Source: CAD feature listing. Evaluate the final solid. Frame: model axes, mm. A direction names the side the tool comes from. Coordinates: 2 decimals unless noted, no trailing zeros. Write each loop counter-clockwise with the first axis right and the second up, starting at its lowest first coordinate (ties: lowest second). Pieces come first, ordered by that corner, then holes. Notation, with made-up numbers: (5.25, -2.5) - (47.25, -2.5) arc R14 cw to (47.25, 1.5) - close; hole circle Ø1 at (22, 66.5). An arc over 180 degrees is marked (long way). One line per question, with ' | ' between items. Start each with the question number.
Q1. Cut plane A-A, the plane y = 14.5. Return loops of the section in (x, z), plus the area to 3 significant figures.
Q2. Draft query along Z for faces 5 (the face through (-20, 51, 15)), 6 (the face through (15, 37, 20)), 7 (the face through (0, 50, 0)), 8 (the face through (12.5, 25, 16)). Return one class per face: +Z half, -Z half, draft (parallel to the pull), parting line (faces both ways), or undercut.
Q3. Access query for faces 1 (the face through (10, 63, -5)), 2 (the face through (-20.5, 25, 0)), 3 (the face through (10.2, 60.5, -7.5)), 4 (the face through (15, 37, -20)). Directions: +Z, -Z, +X, -X, +Y, -Y. A direction counts if a zero-diameter tool reaches every point of the face in a straight line with its end or side. Return the directions, or none.
Q4. Line query: line 1 (X direction, y = 3.5, z = 20); line 2 (X direction, y = 19, z = 0). Output: solid intervals per line, ascending.
Q5. Cut plane C-C, the plane x = -0.5. Return loops of the section in (y, z).
Q6. Contact query for flat-ended pins moving along their axis: P1, Ø5, axis at y = 23.5, z = -18, coming from the +X side; P2, Ø8, axis at x = 21, y = 37.5, coming from the -Z side; P3, Ø2, axis at x = -17.5, z = 4.5, coming from the -Y side; P4, Ø3, axis at y = 20.5, z = 16, coming from the -X side. Output: stop coordinate, or through.
Q7. Cut plane B-B, the plane z = 14. Return loops of the section in (x, y), plus the area to 3 significant figures.
Q8. Cut plane D-D, the plane y = 61. Return loops of the section in (x, z), plus the area to 3 significant figures.
```python
from build123d import *

# Parameters (mm, degrees)
SKETCH1_W           = 50
SKETCH1_H           = 50
BOSS_EXTRUDE1_DEPTH = 64
SKETCH2_W           = 10
SKETCH2_H           = 10
CUT_EXTRUDE1_DEPTH  = 55
CUT_EXTRUDE2_DEPTH  = 30
SKETCH4_W           = 10
SKETCH4_H           = 30
BOSS_EXTRUDE2_DEPTH = 30
SKETCH6_W           = 8
SKETCH6_H           = 25
SKETCH6_W_2         = 25
SKETCH6_H_2         = 8
CUT_EXTRUDE4_DEPTH  = 50
SKETCH7_R           = 3.6
CUT_EXTRUDE5_DEPTH  = 50
SKETCH8_R           = 2.65
CUT_EXTRUDE6_DEPTH  = 50


with BuildPart() as part:
    # Sketch1 → Boss-Extrude1 (new body)
    with BuildSketch(Plane(origin=(0, 0, 0), x_dir=(1, 0, 0), z_dir=(0, 1, 0))):
        Rectangle(SKETCH1_W, SKETCH1_H)
    extrude(amount=BOSS_EXTRUDE1_DEPTH)

    # Sketch2 → Cut-Extrude1 (cut)
    with BuildSketch(Plane(origin=(0, 64, 0), x_dir=(1, 0, 0), z_dir=(0, 1, 0))):
        with Locations((20, 20)):
            Rectangle(SKETCH2_W, SKETCH2_H)
        with Locations((-20, 20)):
            Rectangle(SKETCH2_W, SKETCH2_H)
        with Locations((20, -20)):
            Rectangle(SKETCH2_W, SKETCH2_H)
        with Locations((-20, -20)):
            Rectangle(SKETCH2_W, SKETCH2_H)
    extrude(amount=-CUT_EXTRUDE1_DEPTH, mode=Mode.SUBTRACT)

    # Sketch3 → Cut-Extrude2 (cut)
    with BuildSketch(Plane(origin=(25, 0, 0), x_dir=(0, 0, -1), z_dir=(1, 0, 0))):
        Polygon((-5, 64), (5, 64), (5, 62), (10, 59), (10, 57), (-10, 57), (-10, 59), (-5, 62), align=None)
    extrude(amount=-CUT_EXTRUDE2_DEPTH, mode=Mode.SUBTRACT)

    # Sketch4 → Boss-Extrude2 (add)
    with BuildSketch(Plane(origin=(0, 64, 0), x_dir=(1, 0, 0), z_dir=(0, 1, 0))):
        with Locations((-20, 0)):
            Rectangle(SKETCH4_W, SKETCH4_H)
    extrude(amount=BOSS_EXTRUDE2_DEPTH)

    # Sketch6 → Cut-Extrude4 (cut)
    with BuildSketch(Plane.XZ):
        with Locations((-16.5, 0)):
            Rectangle(SKETCH6_W, SKETCH6_H)
        with Locations((0, 16.5)):
            Rectangle(SKETCH6_W_2, SKETCH6_H_2)
        Rectangle(SKETCH6_W_2, SKETCH6_H)
        with Locations((16.5, 0)):
            Rectangle(SKETCH6_W, SKETCH6_H)
        with Locations((0, -16.5)):
            Rectangle(SKETCH6_W_2, SKETCH6_H_2)
    extrude(amount=-CUT_EXTRUDE4_DEPTH, mode=Mode.SUBTRACT)

    # Sketch7 → Cut-Extrude5 (cut)
    with BuildSketch(Plane(origin=(-15, 0, 0), x_dir=(0, 0, -1), z_dir=(1, 0, 0))):
        with Locations((0, 79.221173682)):
            Circle(SKETCH7_R)
    extrude(amount=-CUT_EXTRUDE5_DEPTH, mode=Mode.SUBTRACT)

    # Sketch8 → Cut-Extrude6 (cut)
    with BuildSketch(Plane(origin=(0, 9, 0), x_dir=(1, 0, 0), z_dir=(0, 1, 0))):
        with Locations(Location((20, -20, 0), (0, 0, 270))):
            Circle(SKETCH8_R)
        with Locations(Location((-20, -20, 0), (0, 0, 270))):
            Circle(SKETCH8_R)
        with Locations(Location((-20, 20, 0), (0, 0, 270))):
            Circle(SKETCH8_R)
        with Locations(Location((20, 20, 0), (0, 0, 270))):
            Circle(SKETCH8_R)
    extrude(amount=-CUT_EXTRUDE6_DEPTH, mode=Mode.SUBTRACT)


solid = part.part
```
Reply:
1) outline: (-25, -15) - (-15, -15) - (-15, -25) - (15, -25) - (15, -15) - (25, -15) - (25, 15) - (15, 15) - (15, 25) - (-15, 25) - (-15, 15) - (-25, 15) - close; hole (-20.5, -12.5) - (-12.5, -12.5) - (-12.5, -20.5) - (12.5, -20.5) - (12.5, -12.5) - (20.5, -12.5) - (20.5, 12.5) - (12.5, 12.5) - (12.5, 20.5) - (-12.5, 20.5) - (-12.5, 12.5) - (-20.5, 12.5) - close | area: 675 mm^2
2) face 5: +Z half | face 6: draft | face 7: undercut | face 8: undercut
3) face 1: +X, +Y | face 2: -Y | face 3: +X | face 4: -Z, +X, +Y
4) line 1: x = -25 to -22.65, -17.35 to -12.5, 12.5 to 17.35, 22.65 to 25 | line 2: x = -25 to -20.5, 20.5 to 25
5) outline: (0, -25) - (64, -25) - (64, -5) - (62, -5) - (59, -10) - (57, -10) - (57, 10) - (59, 10) - (62, 5) - (64, 5) - (64, 25) - (0, 25) - (0, 20.5) - (50, 20.5) - (50, -20.5) - (0, -20.5) - close
6) P1: stops at x = 15 | P2: stops at z = -15 | P3: stops at y = 50 | P4: stops at x = -25
7) outline: (-25, 0) - (-12.5, 0) - (-12.5, 50) - (12.5, 50) - (12.5, 0) - (25, 0) - (25, 64) - (-15, 64) - (-15, 94) - (-25, 94) - close | area: 2,250 mm^2
8) outline: (-25, -15) - (-15, -15) - (-15, -25) - (15, -25) - (15, -15) - (25, -15) - (25, -6.67) - (-5, -6.67) - (-5, 6.67) - (25, 6.67) - (25, 15) - (15, 15) - (15, 25) - (-15, 25) - (-15, 15) - (-25, 15) - close | area: 1,700 mm^2
